```python
from build123d import *

# Parameters (mm, degrees)
SKETCH1_W           = 40
SKETCH1_H           = 40
BOSS_EXTRUDE1_DEPTH = 40
CUT_EXTRUDE1_DEPTH  = 40
SKETCH3_W           = 20
SKETCH3_H           = 20
CUT_EXTRUDE2_DEPTH  = 40
CUT_EXTRUDE3_DEPTH  = 20
SKETCH5_W           = 20
SKETCH5_H           = 20
CUT_EXTRUDE4_DEPTH  = 20


with BuildPart() as part:
    # Sketch1 → Boss-Extrude1 (new body)
    with BuildSketch(Plane.XY):
        with Locations((20, 20)):
            Rectangle(SKETCH1_W, SKETCH1_H)
    extrude(amount=BOSS_EXTRUDE1_DEPTH)

    # Sketch2 → Cut-Extrude1 (cut)
    with BuildSketch(Plane.XY.offset(40)):
        Polygon((40, 40), (0, 20), (0, 40), align=None)
    extrude(amount=-CUT_EXTRUDE1_DEPTH, mode=Mode.SUBTRACT)

    # Sketch3 → Cut-Extrude2 (cut)
    with BuildSketch(Plane(origin=(40, 0, 0), x_dir=(0, 0, -1), z_dir=(1, 0, 0))):
        with Locations((-30, 30)):
            Rectangle(SKETCH3_W, SKETCH3_H)
    extrude(amount=-CUT_EXTRUDE2_DEPTH, mode=Mode.SUBTRACT)

    # Sketch4 → Cut-Extrude3 (cut)
    with BuildSketch(Plane.XZ):
        Polygon((40, 0), (40, 20), (20, 0), align=None)
    extrude(amount=-CUT_EXTRUDE3_DEPTH, mode=Mode.SUBTRACT)

    # Sketch5 → Cut-Extrude4 (cut)
    with BuildSketch(Plane(origin=(0, 20, 0), x_dir=(1, 0, 0), z_dir=(0, 1, 0))):
        with Locations((10, -30)):
            Rectangle(SKETCH5_W, SKETCH5_H)
    extrude(amount=-CUT_EXTRUDE4_DEPTH, mode=Mode.SUBTRACT)


solid = part.part
```
Geometry check sheet. Reference: the model listing, model coordinates, mm. A direction names the side the tool comes from. Coordinates: 2 decimals unless noted, no trailing zeros. Order: outer loops, then holes, each group sorted by start corner. A loop starts at its lowest first (then second) coordinate and runs counter-clockwise, first axis right, second up.
Item 1: Section check B-B (y = 11). Enter the section's corners in (x, z).
Item 2: Depth check by flat-ended pin: pin 1 (8 mm diameter, centred on x = 8, z = 9.5, fed in from +Y); pin 2 (3 mm diameter, centred on y = 16.5, z = 27, fed in from -X); pin 3 (10 mm diameter, centred on x = 30.5, z = 28.5, fed in from +Y); pin 4 (3 mm diameter, centred on x = 25, y = 20, fed in from -Z). Enter the tip coordinate at first touch or a pass-through.
Item 3: Scan lines: line 1 along Z through (x, y) = (34.5, 22); line 2 along X through (y, z) = (2.5, 38). Record each from-to range of solid material in increasing order.
Item 4: Section check C-C (z = 13.5). Enter the section's corners in (x, y).
Item 5: Tool access check on faces 1 (the flat face through (20, 10, 30)), 2 (the flat face through (30, 20, 30)), 3 (the flat face through (30, 10, 40)), 4 (the flat face through (30, 10, 10)). Record the directions out of +Z, -Z, +X, -X, +Y, -Y that give a thin tool (end or side, any length) a straight path to the whole face; none if there is none.
Item 6: Section check A-A (x = 27.5). Enter the section's corners in (y, z).
Item 7: Section check D-D (z = 4). Enter the section's corners in (x, y).
Check sheet entries:
1. outline: (0, 0) - (20, 0) - (40, 20) - (40, 40) - (20, 40) - (20, 20) - (0, 20) - close
2. pin 1: stops at y = 26
2. pin 2: stops at x = 20
2. pin 3: stops at y = 20
2. pin 4: stops at z = 0
3. line 1: z = 0 to 20
3. line 2: x = 20 to 40
4. outline: (0, 0) - (33.5, 0) - (33.5, 20) - (40, 20) - (40, 40) - (0, 20) - close
5. face 1: +Z, -X, +Y, -Y
5. face 2: +Z, +X, -X, +Y
5. face 3: +Z, +X, -X, +Y, -Y
5. face 4: -Z, +X, -Y
6. outline: (0, 7.5) - (20, 7.5) - (20, 0) - (33.75, 0) - (33.75, 20) - (20, 20) - (20, 40) - (0, 40) - close
7. outline: (0, 0) - (24, 0) - (24, 20) - (40, 20) - (40, 40) - (0, 20) - close
